Could you check a few things on this model? Use its own coordinates, in mm. Coordinates: 2 decimals unless noted, no trailing zeros. Loops run counter-clockwise (first coordinate to the right, second up) from the corner with the lowest first, then second, coordinate; pieces in that order, holes last.
1) Thinking about a two-plate mould opening in Y: for faces 1 (the face through (6.358, 41.273, 2.535)), 2 (the face through (10, 50, 2)), 3 (the face through (19, 25, 2)), which applies, released by +Y, released by -Y, zero draft, split by the parting line, or undercut?
2) Imagine slicing it at B-B on x = 6. Please give me the cut outline in (y, z).
3) Imagine slicing it at D-D on z = 4.05. Please give me the cut outline in (x, y), plus the area to 3 significant figures.
4) If I drill on line 1 along Y through (x, z) = (6, 3.5); line 2 along Y through (x, z) = (4.75, 1.1); line 3 along X through (y, z) = (42.5, 2.65), over which ranges is the centre line in solid material (lowest first)?
Autodesk Fusion 360 part; units mm, degrees
sketch "Sketch3" plane through (0, 0, 0) normal (0, 0, 1) x (1, 0, 0)
  line L0 (0, 0) -> (20, 0)
  line L1 (20, 0) -> (20, 50)
  line L2 (20, 50) -> (0, 50)
  line L3 (0, 50) -> (0, 0)
  dimension "d19" = 20
  dimension "d20" = 50
extrude "Extrude1" add sketch "Sketch3" along normal blind 5
fillet "Fillet2" radius 5 1 edges at (20, 25, 0)
sketch "Sketch7" plane through (0, 0, 5) normal (0, 0, 1) x (-1, 0, 0)
  line L0 (0, -50) -> (0, 0)
  line L1 (0, 0) -> (-20, 0)
  line L2 (-20, 0) -> (-20, -50)
  line L3 (-20, -50) -> (0, -50)
  circle A0 centre (-6, -6) radius 2.75
  circle A1 centre (-6, -44) radius 2.75
  dimension "d47" = 5.5
  dimension "d48" = 5.5
  dimension "d49" = 6
  dimension "d50" = 6
  dimension "d51" = 6
  dimension "d52" = 6
extrude "Extrude5" cut sketch "Sketch7" against normal blind 5 contours A0 | A1
Filled in:
1. face 1: undercut
1. face 2: released by +Y
1. face 3: zero draft
2. outline: (0, 0) - (3.25, 0) - (3.25, 5) - (0, 5) - close; (8.75, 0) - (41.25, 0) - (41.25, 5) - (8.75, 5) - close; (46.75, 0) - (50, 0) - (50, 5) - (46.75, 5) - close
3. outline: (0, 0) - (19.91, 0) - (19.91, 50) - (0, 50) - close; hole circle Ø5.5 at (6, 6); hole circle Ø5.5 at (6, 44)
3. area: 948 mm2
4. line 1: y = 0 to 3.25, 8.75 to 41.25, 46.75 to 50
4. line 2: y = 0 to 3.55, 8.45 to 41.55, 46.45 to 50
4. line 3: x = 0 to 3.7, 8.3 to 19.41
